from build123d import *

# Parameters (mm, degrees)
F0_R     = 14.445
F0_R_2   = 12.945
F1_DEPTH = 13
F2_R     = 16.5
F3_DEPTH = 3
F4_R     = 2.99999


# Not quite as in the source:
# - a fillet or chamfer is up to 0.001 mm smaller than in the source, because OpenCascade refuses the exact size


with BuildPart() as f1:
    # F0 (on Top) → F1 (new body)
    with BuildSketch(Plane.XY):
        Circle(F0_R)
        Circle(F0_R_2, mode=Mode.SUBTRACT)
    extrude(amount=F1_DEPTH)

    # F2 (on face) → F3 (join)
    with BuildSketch(Plane.XY.offset(13)):
        Circle(F2_R)
    extrude(amount=F3_DEPTH)

    # F4 (radius 3 in the source; OpenCascade refuses exactly that, so slightly less here)
    f4_edges = [f1.edges().sort_by_distance(p)[0] for p in [
        (-16.5, 0, 16),
        (-12.945, 0, 13),
    ]]
    fillet(f4_edges, radius=F4_R)


solid = f1.part
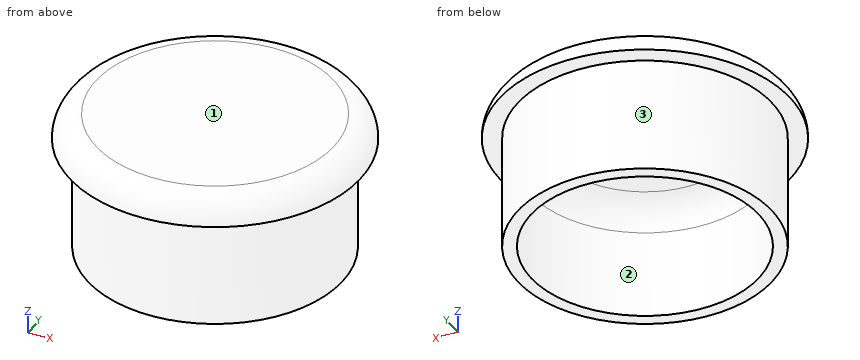
Verification items for the finished model (mm, model axes). Face numbers are marked on the shaded views. Give positions to 0.01 mm unless a question says otherwise; leave off trailing zeros. Order: outer loops, then holes, each group sorted by start corner. A loop starts at its lowest first (then second) coordinate and runs counter-clockwise, first axis right, second up. Notation, with made-up numbers: M -14.5,82.5 L 37.5,82.5 A5 cw 37.5,91.5 Z; hole C 81.25,80 d5. An arc over 180 degrees is marked long. Answer as a JSON object with one key per item and string values. Group by question number.
1) Cross-section at D-D (z = 14.5). Enter the section's corners in (x, y), then the cut area to 3 significant figures.
2) Depth check by flat-ended pin: pin 1 Ø4 at (y, z) = (-7.5, 10.5) entering from -X; pin 2 Ø8 at (x, z) = (8.5, 9.5) entering from +Y; pin 3 Ø3 at (y, z) = (-9.5, 10.5) entering from +X. Enter the tip coordinate at first touch or a pass-through.
3) Cross-section at C-C (z = 3.5). Enter the section's corners in (x, y) (3 decimals).
4) Mould release check, pull along Y, two halves, no side actions. Record for the marked faces 1, 2 and 3: released by +Y, released by -Y, zero draft, split by the parting line, or undercut.
5) Scan lines: line 1 along Y through (x, z) = (0, 6.25) (3 decimals); line 2 along Z through (x, y) = (-2, 6.5); line 3 along X through (y, z) = (-1, 11.5). Record each from-to range of solid material in increasing order. Write a range as [from, to].
Result sheet:
{
 "1": {"outline": "C 0,0 d32.2", "area": "814 mm2"},
 "2": {"pin 1": "stops at x = -13.36", "pin 2": "stops at y = 15.14", "pin 3": "stops at x = 12.03"},
 "3": {"outline": "C 0,0 d28.89; hole C 0,0 d25.89"},
 "4": {"face 1": "zero draft", "face 2": "undercut", "face 3": "split by the parting line"},
 "5": {"line 1": "y = [-14.445, -12.945], [12.945, 14.445]", "line 2": "z = [13, 16]", "line 3": "x = [-14.41, -12.5], [12.5, 14.41]"}
}
